For this review, take the finished solid that the model builds, in its own axes (mm). Give positions to 0.01 mm unless a question says otherwise; leave off trailing zeros. Loops run counter-clockwise (first coordinate to the right, second up) from the corner with the lowest first, then second, coordinate; pieces in that order, holes last.
```python
from build123d import *

# Parameters (mm, degrees)
BOSS_EXTRUDE1_DEPTH = 25.4
SKETCH2_R           = 3.175
CUT_EXTRUDE1_DEPTH  = 25.4


with BuildPart() as part:
    # Sketch1 → Boss-Extrude1 (new body)
    with BuildSketch(Plane.XY):
        with BuildLine():
            Line((-9.010920048, 10.647675717), (-11.233987821, 10.647675717))
            Line((-11.233987821, 10.647675717), (-11.233987821, -8.006537715))
            Line((-11.233987821, -8.006537715), (4.006012179, -8.006537715))
            Line((4.006012179, -8.006537715), (4.006012179, 17.393462285))
            Line((4.006012179, 17.393462285), (-3.613987821, 17.393462285))
            Line((-3.613987821, 17.393462285), (-3.613987821, 16.123462285))
            ThreePointArc((-3.613987821, 16.123462285), (0.23019987, 6.937133014), (-9.010920048, 10.647675717))
        make_face()
    extrude(amount=BOSS_EXTRUDE1_DEPTH)

    # Sketch2 → Cut-Extrude1 (cut)
    with BuildSketch(Plane(origin=(4.006012179, 0, 0), x_dir=(0, 0, -1), z_dir=(1, 0, 0))):
        with Locations(Location((-19.05, -1.656537715, 0), (0, 0, 90))):
            Circle(SKETCH2_R)
        with Locations(Location((-6.35, -1.656537715, 0), (0, 0, 90))):
            Circle(SKETCH2_R)
    extrude(amount=-CUT_EXTRUDE1_DEPTH, mode=Mode.SUBTRACT)


solid = part.part
```
Q1. Mouldability with a two-part tool opening along Y and no side actions: class faces 1 (the flat face through (-10, 10.648, 13)), 2 (the flat face through (-3.614, 17, 13)), 3 (the cylindrical face through (-3.507, 0.05, 9.027)) as +Y half, -Y half, draft (parallel to the pull), parting line (faces both ways), or undercut.
Answers:
face 1: +Y half
face 2: draft
face 3: undercut
Q2. Consider section D-D on x = -7.5. Give the boundary of the cut face in (y, z) (3 decimals).
Answers:
outline: (-8.007, 0) - (6.98, 0) - (6.98, 25.4) - (-8.007, 25.4) - close; hole circle Ø6.35 at (-1.657, 6.35); hole circle Ø6.35 at (-1.657, 19.05)
Q3. Consider section C-C on z = 11.5. Give the boundary of the cut face in (x, y) (1 decimal), plus the area to 3 significant figures.
Answers:
outline: (-11.2, -8) - (4, -8) - (4, 17.4) - (-3.6, 17.4) - (-3.6, 16.1) arc R5.4 cw (long way) to (-9, 10.6) - (-11.2, 10.6) - close
area: 267 mm2
Q4. For pin 1 Ø1.1 at (x, z) = (-10, 16) entering from +Y, flat-tipped, find the tip position at first contact; note if it passes through.
Answers:
pin 1: stops at y = 10.65
Q5. Consider section B-B on y = -0.5. Give the boundary of the cut face in (x, z).
Answers:
outline: (-11.23, 0) - (4.01, 0) - (4.01, 3.39) - (-11.23, 3.39) - close; (-11.23, 9.31) - (4.01, 9.31) - (4.01, 16.09) - (-11.23, 16.09) - close; (-11.23, 22.01) - (4.01, 22.01) - (4.01, 25.4) - (-11.23, 25.4) - close
Q6. For probe 1 along Z at (x, y) = (-6.5, -1.75); probe 2 along Y at (x, z) = (-2.5, 16.5); probe 3 along Z at (x, y) = (-4, -0.75), list the stretches that pass through material, from the lowest coordinate up.
Answers:
probe 1: z = 0 to 3.18, 9.52 to 15.88, 22.22 to 25.4
probe 2: y = -8.01 to -3.55, 0.24 to 5.44, 16.01 to 17.39
probe 3: z = 0 to 3.31, 9.39 to 16.01, 22.09 to 25.4
Q7. Consider section A-A on z = 19.05. Give the boundary of the cut face in (x, y) (1 decimal), plus the area to 3 significant figures.
Answers:
outline: (-11.2, -8) - (4, -8) - (4, -4.8) - (-11.2, -4.8) - close; (-11.2, 1.5) - (4, 1.5) - (4, 17.4) - (-3.6, 17.4) - (-3.6, 16.1) arc R5.4 cw (long way) to (-9, 10.6) - (-11.2, 10.6) - close
area: 171 mm2
